For this review, use the dimensioned drawing (mm, ordinates from the lowest corner) and the shaded views. A direction names the side the tool comes from. Coordinates: 2 decimals unless noted, no trailing zeros. Loops run counter-clockwise (first coordinate to the right, second up) from the corner with the lowest first, then second, coordinate; pieces in that order, holes last. Notation, with made-up numbers: M 18.5,71.5 L 39.5,71.5 A10 cw 39.5,80.5 Z; hole C 19.5,48 d2. An arc over 180 degrees is marked long. One line per item, written item: value.
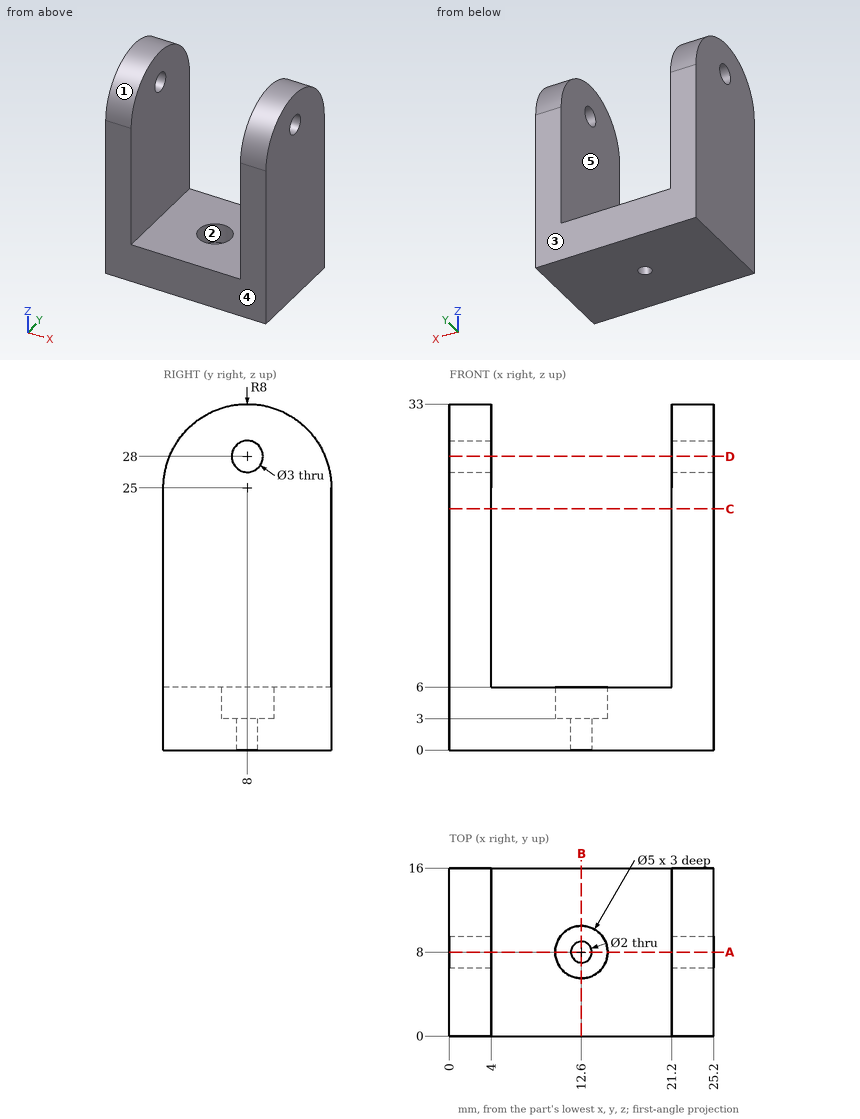
(1) Add section A-A on y = 8. State the section outline as (x, z) points.
Checks:
outline: M 0,0 L 11.6,0 L 11.6,3 L 10.1,3 L 10.1,6 L 4,6 L 4,26.5 L 0,26.5 Z; M 0,29.5 L 4,29.5 L 4,33 L 0,33 Z; M 13.6,0 L 25.2,0 L 25.2,26.5 L 21.2,26.5 L 21.2,6 L 15.1,6 L 15.1,3 L 13.6,3 Z; M 21.2,29.5 L 25.2,29.5 L 25.2,33 L 21.2,33 Z
(2) To check wall thickness, follow L1, parallel to X at y = 13.5, z = 18; L2, parallel to Y at x = 12.6, z = 1.15; L3, parallel to Z at x = 23.3, y = 8. State the ranges of each line that lie inside material, in increasing order. Write a range as [from, to].
Checks:
L1: [0, 4], [21.2, 25.2]
L2: [0, 7], [9, 16]
L3: [0, 26.5], [29.5, 33]
(3) Add section B-B on x = 12.6. State the section outline as (y, z) points.
Checks:
outline: M 0,0 L 7,0 L 7,3 L 5.5,3 L 5.5,6 L 0,6 Z; M 9,0 L 16,0 L 16,6 L 10.5,6 L 10.5,3 L 9,3 Z
(4) Insertion check: pin 1 Ø1.8 at (x, y) = (12.6, 8) entering from +Z; pin 2 Ø3 at (x, y) = (6, 8) entering from +Z; pin 3 Ø4 at (x, y) = (12.6, 8) entering from +Z. Each pin has a flat end and moves straight along its axis. Give the tip position at first contact, or say it passes through.
Checks:
pin 1: through
pin 2: z = 6
pin 3: z = 3
(5) Add section D-D on z = 28. State the section outline as (x, y) points.
Checks:
outline: M 0,0.58 L 4,0.58 L 4,6.5 L 0,6.5 Z; M 0,9.5 L 4,9.5 L 4,15.42 L 0,15.42 Z; M 21.2,0.58 L 25.2,0.58 L 25.2,6.5 L 21.2,6.5 Z; M 21.2,9.5 L 25.2,9.5 L 25.2,15.42 L 21.2,15.42 Z
(6) Tool access review of the marked faces 4 and 5: name each direction out of +Z, -Z, +X, -X, +Y, -Y from which nothing blocks a thin tool from reaching the whole face with its end or side.
Checks:
face 4: +Z, -Z, +X, -X, -Y
face 5: +Z, +Y, -Y
(7) Add section C-C on z = 23. State the section outline as (x, y) points, then the cut area to 3 significant figures.
Checks:
outline: M 0,0 L 4,0 L 4,16 L 0,16 Z; M 21.2,0 L 25.2,0 L 25.2,16 L 21.2,16 Z
area: 128 mm^2
(8) Draft analysis for pull direction Y (two halves, no side actions). For the marked faces 1, 2 and 3, state which applies: pulls with the +Y half, pulls with the -Y half, needs draft (parallel to the pull), parting line crosses it, or undercut.
Checks:
face 1: parting line crosses it
face 2: undercut
face 3: pulls with the +Y half
